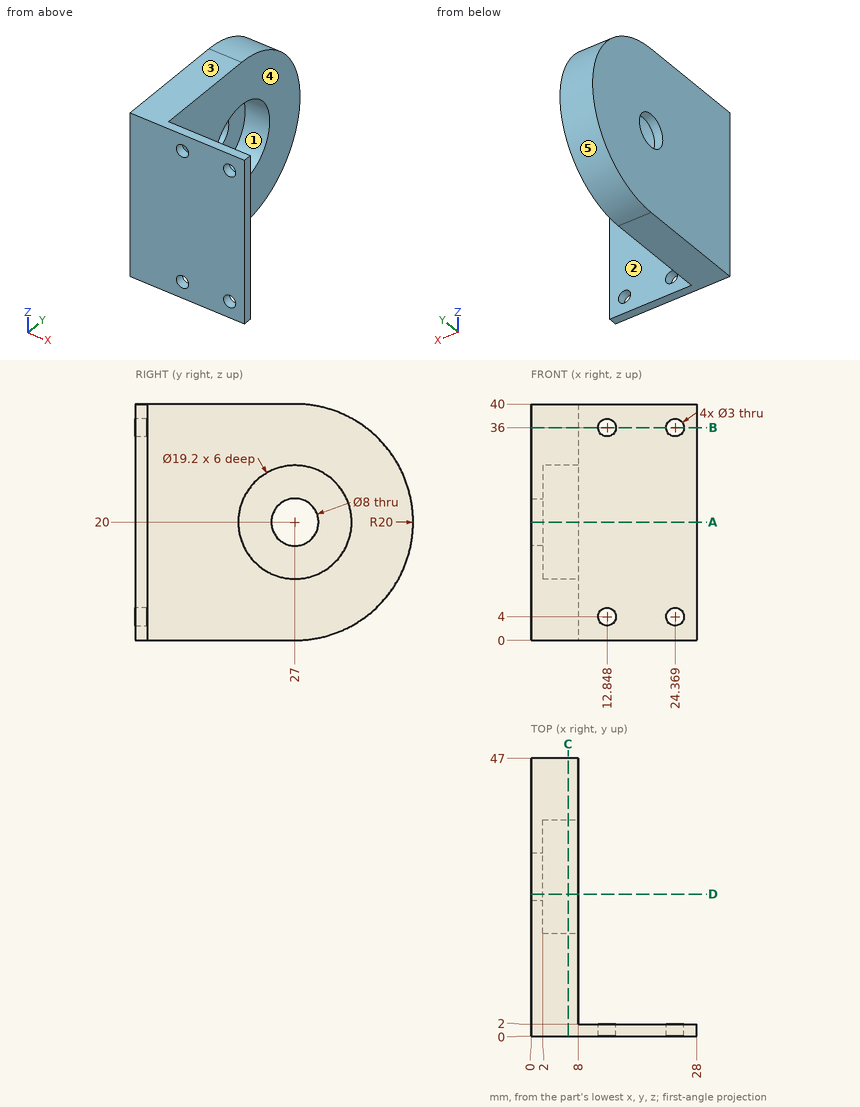
The drawing under review shows one solid part. Ordinate dimensions are in mm from its lowest x, y, z. A direction names the side the tool comes from. Coordinates: 2 decimals unless noted, no trailing zeros. Write each loop counter-clockwise with the first axis right and the second up, starting at its lowest first coordinate (ties: lowest second). Pieces come first, ordered by that corner, then holes.
1) Add section B-B (z = 36). Write out the cut boundary in (x, y).
2) Add section D-D (y = 24). Write out the cut boundary in (x, z).
3) To check wall thickness, follow L1, parallel to X at y = 1.55, z = 36; L2, parallel to Y at x = 4.05, z = 20; L3, parallel to Y at x = 16.5, z = 3. State the ranges of each line that lie inside material, in increasing order.
4) Add section A-A (z = 20). Write out the cut boundary in (x, y), plus the area to 3 significant figures.
5) Add section C-C (x = 6.25). Write out the cut boundary in (y, z), plus the area to 3 significant figures.
6) Mouldability with a two-part tool opening along Z and no side actions: class the marked faces 1, 2 and 3 as +Z half, -Z half, draft (parallel to the pull), parting line (faces both ways), or undercut.
7) Insertion check: pin 1 (1 mm diameter, centred on y = 15, z = 32, fed in from -X); pin 2 (6 mm diameter, centred on y = 31.5, z = 20.5, fed in from +X); pin 3 (5 mm diameter, centred on y = 11.5, z = 7, fed in from +X); pin 4 (6 mm diameter, centred on x = 14.5, z = 20, fed in from +Y). Each pin has a flat end and moves straight along its axis. Give the tip position at first contact, or say it passes through.
8) Machinability: for the marked faces 4 and 5, which of the approach directions +Z, -Z, +X, -X, +Y, -Y give a long, thin tool a straight path to every point of the face, cutting with its end or side? Answer none if there is none.
Check result:
1. outline: (0, 0) - (11.35, 0) - (11.35, 2) - (8, 2) - (8, 39) - (0, 39) - close; (14.35, 0) - (22.87, 0) - (22.87, 2) - (14.35, 2) - close; (25.87, 0) - (28, 0) - (28, 2) - (25.87, 2) - close
2. outline: (0, 0) - (8, 0) - (8, 10.88) - (2, 10.88) - (2, 17.35) - (0, 17.35) - close; (0, 22.65) - (2, 22.65) - (2, 29.12) - (8, 29.12) - (8, 40) - (0, 40) - close
3. L1: x = 0 to 11.35, 14.35 to 22.87, 25.87 to 28
3. L2: y = 0 to 17.4, 36.6 to 47
3. L3: y = 0 to 2
4. outline: (0, 0) - (28, 0) - (28, 2) - (8, 2) - (8, 17.4) - (2, 17.4) - (2, 23) - (0, 23) - close; (0, 31) - (2, 31) - (2, 36.6) - (8, 36.6) - (8, 47) - (0, 47) - close
4. area: 285 mm2
5. outline: (0, 0) - (27, 0) arc R20 ccw to (27, 40) - (0, 40) - close; hole circle Ø19.2 at (27, 20)
5. area: 1,420 mm2
6. face 1: undercut
6. face 2: draft
6. face 3: +Z half
7. pin 1: stops at x = 0
7. pin 2: stops at x = 2
7. pin 3: stops at x = 8
7. pin 4: stops at y = 2
8. face 4: +Z, -Z, +X, +Y
8. face 5: +X, -X, +Y
